```python
from build123d import *

# Parameters (mm, degrees)
PAD_DEPTH     = 3
SKETCH002_R   = 2.75
PAD002_DEPTH  = 2
CHAMFER_SIZE2 = 1.99
CHAMFER_SIZE  = 1.5
SKETCH005_R   = 1.55
POCKET_DEPTH  = 5


with BuildPart() as part:
    # Sketch → Pad (new body)
    with BuildSketch(Plane.XY):
        with BuildLine():
            Line((0, 64.75), (0, 31.219))
            add(Edge.make_bspline(
                [(0, 31.219), (0, 0), (16.1875, 0), (18.5, 0)],
                knots=[0, 0, 0, 0, 1, 1, 1, 1], degree=3))
            Line((18.5, 0), (74, 0))
            add(Edge.make_bspline(
                [(74, 0), (78.625, 0), (78.625, 8.09375), (83.25, 8.09375)],
                knots=[0, 0, 0, 0, 1, 1, 1, 1], degree=3))
            Line((83.25, 8.09375), (107.531, 8.09375))
            add(Edge.make_bspline(
                [(107.531, 8.09375), (115.62475, 8.09375), (111.031, 27.74975), (115.656, 27.74975)],
                knots=[0, 0, 0, 0, 1, 1, 1, 1], degree=3))
            Line((115.656, 27.74975), (129.531, 27.74975))
            add(Edge.make_bspline(
                [(129.531, 27.74975), (137.5935, 27.74975), (137.5935, 60.125), (137.5935, 64.75)],
                knots=[0, 0, 0, 0, 1, 1, 1, 1], degree=3))
            ThreePointArc((137.5935, 64.75), (137.254842, 65.567592), (136.43725, 65.90625))
            Line((136.43725, 65.90625), (1.15625, 65.90625))
            ThreePointArc((1.15625, 65.90625), (0.338658, 65.567592), (0, 64.75))
        make_face()
    extrude(amount=PAD_DEPTH)

    # Sketch002 (on Face13 of Pad) → Pad002 (join)
    with BuildSketch(Plane.XY.offset(3)):
        with Locations((9.15, 10.831)):
            Circle(SKETCH002_R)
        with Locations((132.869, 61.281)):
            Circle(SKETCH002_R)
    extrude(amount=PAD002_DEPTH)

    # Chamfer
    chamfer_edges = [part.edges().sort_by_distance(p)[0] for p in [
        (6.4, 10.831, 3),
        (130.119, 61.281, 3),
    ]]
    chamfer_side = part.faces().sort_by_distance((63.310609, 35.968212, 3))[0]
    chamfer(chamfer_edges, length=CHAMFER_SIZE, length2=CHAMFER_SIZE2, reference=chamfer_side)

    # Sketch005 (on Face18 of Chamfer) → Pocket (cut)
    with BuildSketch(Plane.XY.offset(5)):
        with Locations((9.15, 10.831)):
            Circle(SKETCH005_R)
        with Locations((132.869, 61.281)):
            Circle(SKETCH005_R)
    extrude(amount=-POCKET_DEPTH, mode=Mode.SUBTRACT)


solid = part.part
```
For this review, take the finished solid that the model builds, in its own axes (mm). A direction names the side the tool comes from. Coordinates: 2 decimals unless noted, no trailing zeros. Write each loop counter-clockwise with the first axis right and the second up, starting at its lowest first coordinate (ties: lowest second). Pieces come first, ordered by that corner, then holes. Notation, with made-up numbers: (83.5, 30) - (95.5, 30) arc R24 ccw to (95.5, 58) - close; hole circle Ø7 at (60, -39.5). An arc over 180 degrees is marked (long way). Put each result on its own line as item: value.
1. Wall thickness on probe 1 along Z at (x, y) = (38, 31); probe 2 along X at (y, z) = (12, 2.65); probe 3 along X at (y, z) = (39, 2.4): over which ranges is each line inside the solid? List them lowest first.
Values found:
probe 1: 0 to 3
probe 2: 3.01 to 8.13, 10.17 to 111.88
probe 3: 0 to 135.77
2. For pin 1 (0.9 mm diameter, centred on x = 123, z = 1, fed in from -Y); pin 2 (2.5 mm diameter, centred on x = 89.5, z = 2, fed in from -Y); pin 3 (6 mm diameter, centred on x = 85, y = 41, fed in from +Z), all flat-tipped, find the tip position at first contact; note any pin that passes through.
Values found:
pin 1: y = 27.75
pin 2: y = 8.09
pin 3: z = 3
3. Add section A-A, the plane x = 92.5. Give the boundary of the cut face in (y, z).
Values found:
outline: (8.09, 0) - (65.91, 0) - (65.91, 3) - (8.09, 3) - close
4. Add section B-B, the plane x = 56. Give the boundary of the cut face in (y, z).
Values found:
outline: (0, 0) - (65.91, 0) - (65.91, 3) - (0, 3) - close
5. Mouldability with a two-part tool opening along X and no side actions: class faces 3 (the flat face through (0, 48, 1)), 4 (the cylindrical face through (131.32, 61.35, 2.54)), 5 (the flat face through (68, 33, 0)) as released by +X, released by -X, zero draft, split by the parting line, or undercut.
Values found:
face 3: released by -X
face 4: undercut
face 5: zero draft
6. Machinability: for faces 1 (the flat face through (95, 8.094, 1)), 2 (the flat face through (134, 60, 5)), which of the approach directions +Z, -Z, +X, -X, +Y, -Y give a long, thin tool a straight path to every point of the face, cutting with its end or side? Answer none if there is none.
Values found:
face 1: +Z, -Z, +X, -Y
face 2: +Z, +X, -X, +Y, -Y
